Input: part model. Units: mm. Frame: model coordinates. A direction names the side the tool comes from. Give positions to 0.01 mm unless a question says otherwise; leave off trailing zeros. Loops run counter-clockwise (first coordinate to the right, second up) from the corner with the lowest first, then second, coordinate; pieces in that order, holes last. Notation, with made-up numbers: M 24.5,-9 L 76.5,-9 A13 ccw 76.5,-5 Z; hole C 80.25,40 d4. An arc over 180 degrees is marked long. Answer as a JSON object with one key per item and string values. Group by question number.
1) Section query A-A on y = 6. Return loops of the section in (x, z).
2) Section query C-C on z = 21. Return loops of the section in (x, y).
3) First-contact query: P1, Ø1, axis at x = -14, z = 39, coming from the +Y side; P2, Ø5, axis at y = 4, z = -31, coming from the +X side. Flat tips, straight axial feed; report the tip coordinate or a pass-through.
4) Access query for faces 1 (the flat face through (0, 7, 39)), 2 (the flat face through (0, 6, 36)), 3 (the flat face through (-32.32, 4.93, -0.56)). Directions: +Z, -Z, +X, -X, +Y, -Y. A direction counts if a zero-diameter tool reaches every point of the face in a straight line with its end or side. Return the directions, or none.
5) Draft query along Z for faces 4 (the flat face through (0, 5, 37)), 5 (the flat face through (-1, 0, -1)), 6 (the flat face through (-1, 3, 40)). Return one class per face: +Z half, -Z half, draft (parallel to the pull), parting line (faces both ways), or undercut.
6) Ray query, L1, parallel to Z at x = -25, y = 5.25; L2, parallel to Z at x = 12, y = 9.25; L3, parallel to X at y = 3.5, z = 2.5. Return the intervals inside material, ascending.
7) Section query B-B on x = 14. Return loops of the section in (y, z), plus the area to 3 significant figures.
from build123d import *

# Parameters (mm, degrees)
SKETCH1_W           = 74.5
SKETCH1_H           = 80
BOSS_EXTRUDE1_DEPTH = 10
SKETCH2_W           = 11
SKETCH2_H           = 3
CUT_EXTRUDE1_DEPTH  = 75.5
SKETCH3_W           = 2
SKETCH3_H           = 2
CUT_EXTRUDE2_DEPTH  = 75.5
CUT_EXTRUDE4_DEPTH  = 81


with BuildPart() as part:
    # Sketch1 → Boss-Extrude1 (new body)
    with BuildSketch(Plane(origin=(0, 0, 0), x_dir=(1, 0, 0), z_dir=(0, 1, 0))):
        Rectangle(SKETCH1_W, SKETCH1_H)
    extrude(amount=BOSS_EXTRUDE1_DEPTH)

    # Sketch2 → Cut-Extrude1 (cut, through all)
    with BuildSketch(Plane.ZY.offset(37.25)):
        with Locations((34.5, 8.5)):
            Rectangle(SKETCH2_W, SKETCH2_H)
    extrude(amount=-CUT_EXTRUDE1_DEPTH, mode=Mode.SUBTRACT)

    # Sketch3 → Cut-Extrude2 (cut, through all)
    with BuildSketch(Plane.ZY.offset(37.25)):
        with Locations((37, 6)):
            Rectangle(SKETCH3_W, SKETCH3_H)
    extrude(amount=-CUT_EXTRUDE2_DEPTH, mode=Mode.SUBTRACT)

    # Sketch4 → Cut-Extrude4 (cut, through all)
    with BuildSketch(Plane(origin=(0, 0, -40), x_dir=(-1, 0, 0), z_dir=(0, 0, -1))):
        Polygon((-37.25, 0), (-27.25, 10), (-37.25, 10), align=None)
        Polygon((37.25, 10), (37.25, 0), (27.25, 10), align=None)
    extrude(amount=-CUT_EXTRUDE4_DEPTH, mode=Mode.SUBTRACT)


solid = part.part
Output:
{
 "1": {"outline": "M -31.25,-40 L 31.25,-40 L 31.25,36 L -31.25,36 Z; M -31.25,38 L 31.25,38 L 31.25,40 L -31.25,40 Z"},
 "2": {"outline": "M -37.25,0 L 37.25,0 L 27.25,10 L -27.25,10 Z"},
 "3": {"P1": "stops at y = 7", "P2": "stops at x = 35.75"},
 "4": {"face 1": "+Z, +X, -X, +Y", "face 2": "+X, -X, +Y", "face 3": "+Z, -Z, -X, +Y"},
 "5": {"face 4": "undercut", "face 5": "draft", "face 6": "+Z half"},
 "6": {"L1": "z = -40 to 36, 38 to 40", "L2": "z = -40 to 29", "L3": "x = -33.75 to 33.75"},
 "7": {"outline": "M 0,-40 L 10,-40 L 10,29 L 7,29 L 7,36 L 5,36 L 5,38 L 7,38 L 7,40 L 0,40 Z", "area": "763 mm^2"}
}
